```python
from build123d import *

# Parameters (mm, degrees)
BOSS_EXTRUDE1_DEPTH   = 3.175
F_8_32_TAPPED_HOLE1_D = 3.4544
FILLET1_R             = 19.05


with BuildPart() as part:
    # Sketch1 → Boss-Extrude1 (new, symmetric)
    with BuildSketch(Plane(origin=(0, 0, 0), x_dir=(0, 0, -1), z_dir=(1, 0, 0))):
        Polygon((0, 0), (0, 6.35), (-12.7, 6.35), (-12.7, 0), (-25.4, 0), (-25.4, 6.35), (-38.1, 6.35), (-38.1, 0), (-50.8, 0), (-50.8, 6.35), (-63.5, 6.35), (-63.5, -19.05), (0, -19.05), align=None)
    extrude(amount=BOSS_EXTRUDE1_DEPTH, both=True)

    # #8-32 Tapped Hole1 (through all)
    with Locations(Plane(origin=(3.175, 0, 0), x_dir=(0, 0, -1), z_dir=(1, 0, 0))):
        with Locations((-12.7, -9.525), (-25.4, -9.525)):
            Hole(F_8_32_TAPPED_HOLE1_D / 2)

    # Fillet1
    fillet1_edges = [part.edges().sort_by_distance(p)[0] for p in [
        (0, -19.05, 0),
        (0, -19.05, 63.5),
    ]]
    fillet(fillet1_edges, radius=FILLET1_R)


solid = part.part
```
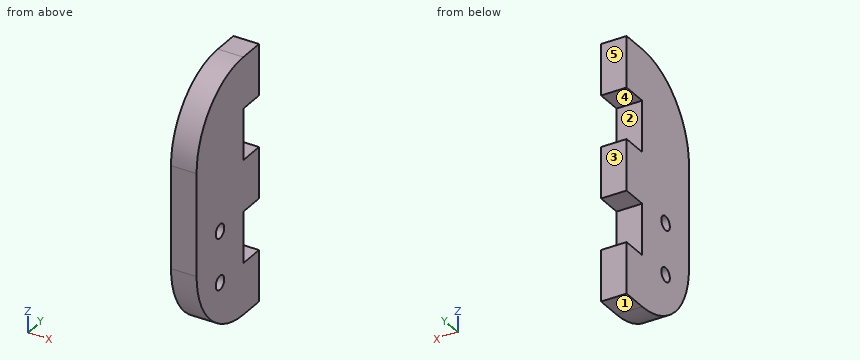
For this review, take the finished solid that the model builds, in its own axes (mm). Face numbers are marked on the shaded views. A direction names the side the tool comes from. Give positions to 0.01 mm unless a question says otherwise; leave off trailing zeros. Write each loop counter-clockwise with the first axis right and the second up, starting at its lowest first coordinate (ties: lowest second). Pieces come first, ordered by that corner, then holes.
Item 1: The part is to be moulded in two halves that separate along Z. For the marked faces 1, 2 and 3, say which applies: +Z half, -Z half, draft (parallel to the pull), parting line (faces both ways), or undercut.
Item 2: Take a section at A-A (x = 1.5). Give the boundary of the cut face in (y, z) (3 decimals).
Item 3: Wall thickness on probe 1 along Z at (x, y) = (-1.5, 5); probe 2 along Z at (x, y) = (1, -8.5); probe 3 along Y at (x, z) = (-1, 4.5): over which ranges is each line inside the solid? List them lowest first.
Item 4: Take a section at C-C (y = -17). Give the boundary of the cut face in (x, z) (3 decimals), and give its area (3 significant figures).
Item 5: Insertion check: P1, Ø1.5, axis at x = 2, y = -13, coming from the +Z side; P2, Ø1.9, axis at x = -1.5, z = 17.5, coming from the +Y side; P3, Ø1.5, axis at x = -2, y = -3, coming from the -Z side. Each pin has a flat end and moves straight along its axis. Give the tip position at first contact, or say it passes through.
Item 6: Machinability: for the marked faces 4 and 5, which of the approach directions +Z, -Z, +X, -X, +Y, -Y give a long, thin tool a straight path to every point of the face, cutting with its end or side? Answer none if there is none.
Item 7: Take a section at B-B (z = 8). Give the boundary of the cut face in (x, y) (3 decimals).
Established:
1. face 1: -Z half
1. face 2: undercut
1. face 3: draft
2. outline: (-19.05, 19.05) arc R19.05 ccw to (0, 0) - (6.35, 0) - (6.35, 12.7) - (0, 12.7) - (0, 25.4) - (6.35, 25.4) - (6.35, 38.1) - (0, 38.1) - (0, 50.8) - (6.35, 50.8) - (6.35, 63.5) - (0, 63.5) arc R19.05 ccw to (-19.05, 44.45) - close; hole circle Ø3.454 at (-9.525, 12.7); hole circle Ø3.454 at (-9.525, 25.4)
3. probe 1: z = 0 to 12.7, 25.4 to 38.1, 50.8 to 63.5
3. probe 2: z = 2 to 11.31, 14.09 to 24.01, 26.79 to 61.5
3. probe 3: y = -12.3 to 6.35
4. outline: (-3.175, 10.453) - (3.175, 10.453) - (3.175, 53.047) - (-3.175, 53.047) - close
4. area: 270 mm2
5. P1: stops at z = 59.04
5. P2: stops at y = 0
5. P3: stops at z = 0.13
6. face 4: +X, -X, +Y
6. face 5: +Z, -Z, +X, -X, +Y
7. outline: (-3.175, -15.518) - (3.175, -15.518) - (3.175, 6.35) - (-3.175, 6.35) - close
